from build123d import *

# Parameters (mm, degrees)
SKETCH1_W           = 101.6
SKETCH1_H           = 36.999999914
BOSS_EXTRUDE1_DEPTH = 5.334
SKETCH2_R           = 15.499999988
MOTORHOLES_DEPTH    = 55.326251062
SKETCH3_W           = 19.05
SKETCH3_H           = 5.334
SKETCH3_H_2         = 5.334001831
BOTTOMTEETH_DEPTH   = 5.334
SKETCH4_W           = 10.668
SKETCH4_H           = 12.7
SIDECUT_DEPTH       = 57.36622313
SKETCH5_W           = 19.05
SKETCH5_H           = 5.334
TOPTEETH_DEPTH      = 21.336


with BuildPart() as part:
    # Sketch1 → Boss-Extrude1 (new body)
    with BuildSketch(Plane.XY):
        Rectangle(SKETCH1_W, SKETCH1_H)
    extrude(amount=BOSS_EXTRUDE1_DEPTH)

    # Sketch2 → MotorHoles (cut, through all)
    with BuildSketch(Plane.XY.offset(5.334)):
        Circle(SKETCH2_R)
    extrude(amount=-MOTORHOLES_DEPTH, mode=Mode.SUBTRACT)

    # Sketch3 → BottomTeeth (add)
    with BuildSketch(Plane.XZ.offset(18.499999957)):
        with Locations((-41.275, 2.667)):
            Rectangle(SKETCH3_W, SKETCH3_H)
        with Locations((41.275, 2.667)):
            Rectangle(SKETCH3_W, SKETCH3_H)
        with Locations((0, 2.667000916)):
            Rectangle(SKETCH3_W, SKETCH3_H_2)
    extrude(amount=BOTTOMTEETH_DEPTH)

    # Sketch4 → SideCut (cut, through all)
    with BuildSketch(Plane.XY.offset(5.334)):
        with Locations((-50.8, 0)):
            Rectangle(SKETCH4_W, SKETCH4_H)
        with Locations((50.8, 0)):
            Rectangle(SKETCH4_W, SKETCH4_H)
    extrude(amount=-SIDECUT_DEPTH, mode=Mode.SUBTRACT)

    # Sketch5 → TopTeeth (add)
    with BuildSketch(Plane(origin=(0, 18.499999957, 0), x_dir=(1, 0, 0), z_dir=(0, 1, 0))):
        with Locations((-41.275, -2.667)):
            Rectangle(SKETCH5_W, SKETCH5_H)
        with Locations((0, -2.667)):
            Rectangle(SKETCH5_W, SKETCH5_H)
    extrude(amount=TOPTEETH_DEPTH)


solid = part.part
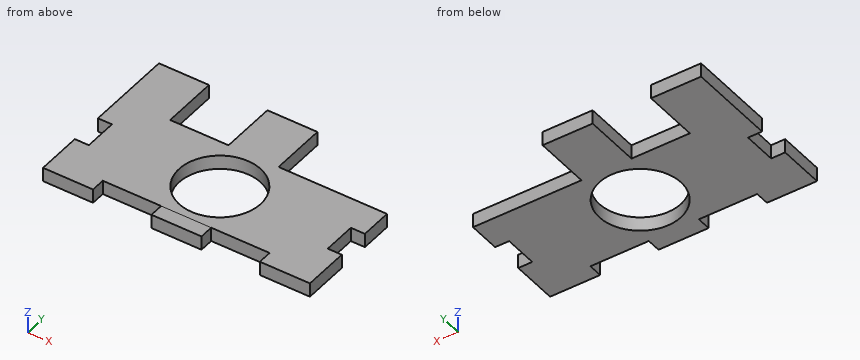
Design review of the part built by this model. Coordinates are the model's own, in mm. Coordinates: 2 decimals unless noted, no trailing zeros. Order: outer loops, then holes, each group sorted by start corner. A loop starts at its lowest first (then second) coordinate and runs counter-clockwise, first axis right, second up. Notation, with made-up numbers: M -13,34.5 L 42,34.5 A7 cw 42,45.5 Z; hole C -35.75,31.5 d6. An arc over 180 degrees is marked long. Use a Markdown table: item, result.
(1) Add section C-C (z = 2.8). Give the boundary of the cut face in (x, y) (3 decimals), then the cut area to 3 significant figures.
Worked answers:
| item | result |
|---|---|
| outline | M -50.8,-23.834 L -31.75,-23.834 L -31.75,-18.5 L -9.525,-18.5 L -9.525,-23.834 L 9.525,-23.834 L 9.525,-18.5 L 31.75,-18.5 L 31.75,-23.834 L 50.8,-23.834 L 50.8,-6.35 L 45.466,-6.35 L 45.466,6.35 L 50.8,6.35 L 50.8,18.5 L 9.525,18.5 L 9.525,39.836 L -9.525,39.836 L -9.525,18.5 L -31.75,18.5 L -31.75,39.836 L -50.8,39.836 L -50.8,6.35 L -45.466,6.35 L -45.466,-6.35 L -50.8,-6.35 Z; hole C 0,0 d31 |
| area | 3,990 mm2 |
(2) Add section A-A (y = 27.5). Give the boundary of the cut face in (x, z) (3 decimals).
Worked answers:
| item | result |
|---|---|
| outline | M -50.8,0 L -31.75,0 L -31.75,5.334 L -50.8,5.334 Z; M -9.525,0 L 9.525,0 L 9.525,5.334 L -9.525,5.334 Z |
(3) Wall thickness on probe 1 along X at (y, z) = (35, 2.9) (3 decimals); probe 2 along Y at (x, z) = (0, 3.1); probe 3 along Y at (x, z) = (-46, 3.8): over which ranges is each line inside the solid? List them lowest first.
Worked answers:
| item | result |
|---|---|
| probe 1 | x = -50.8 to -31.75, -9.525 to 9.525 |
| probe 2 | y = -23.83 to -15.5, 15.5 to 39.84 |
| probe 3 | y = -23.83 to -6.35, 6.35 to 39.84 |
(4) Add section D-D (y = 3.5). Give the boundary of the cut face in (x, z), then the cut area to 3 significant figures.
Worked answers:
| item | result |
|---|---|
| outline | M -45.47,0 L -15.1,0 L -15.1,5.33 L -45.47,5.33 Z; M 15.1,0 L 45.47,0 L 45.47,5.33 L 15.1,5.33 Z |
| area | 324 mm2 |
(5) For P1, Ø2.5, axis at y = 1.5, z = 3, coming from the -X side; P2, Ø2.5, axis at y = 24, z = 3.5, coming from the +X side (3 decimals); P3, Ø1, axis at x = 35, z = 0.5, coming from the +Y side; P4, Ø18.5, axis at x = 0, y = 0, coming from the +Z side, all flat-tipped, find the tip position at first contact; note any pin that passes through.
Worked answers:
| item | result |
|---|---|
| P1 | stops at x = -45.47 |
| P2 | stops at x = 9.525 |
| P3 | stops at y = 18.5 |
| P4 | passes through |
